```python
from build123d import *

# Parameters (mm, degrees)
F0_R     = 6
F1_DEPTH = 2
F2_R     = 2.5
F3_DEPTH = 1
F4_W     = 2.0085166757
F4_H     = 2
F5_DEPTH = 12.5
F6_R     = 0.5


with BuildPart() as f1:
    # F0 (on Front) → F1 (new body)
    with BuildSketch(Plane.XZ):
        Circle(F0_R)
    extrude(amount=F1_DEPTH)

    # F2 (on face) → F3 (cut)
    with BuildSketch(Plane(origin=(0, 0, 0), x_dir=(-1, 0, 0), z_dir=(0, 1, 0))):
        Circle(F2_R)
    extrude(amount=-F3_DEPTH, mode=Mode.SUBTRACT)

    # F4 (on Right) → F5 (cut, symmetric)
    with BuildSketch(Plane.YZ):
        with Locations((-2.1042583379, 0)):
            Rectangle(F4_W, F4_H)
    extrude(amount=F5_DEPTH, both=True, mode=Mode.SUBTRACT)

    # F6
    f6_edges = [f1.edges().sort_by_distance(p)[0] for p in [
        (0, -2, -6),
        (0, -2, 6),
    ]]
    fillet(f6_edges, radius=F6_R)


solid = f1.part
```
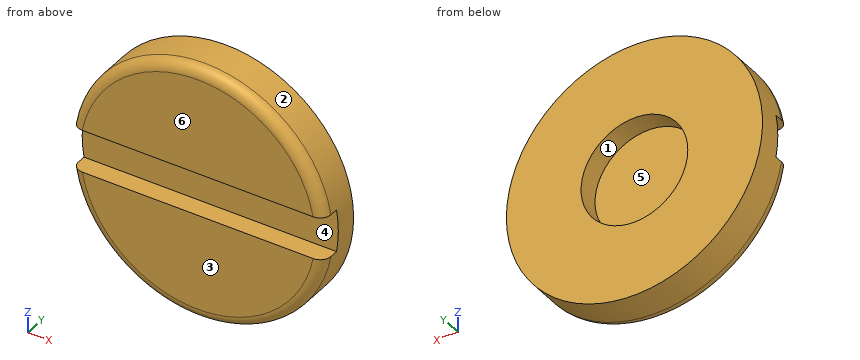
Work out the finished part from the listing and answer in its coordinate system (mm). Face numbers are marked on the shaded views. A direction names the side the tool comes from. Coordinates: 2 decimals unless noted, no trailing zeros. Loops run counter-clockwise (first coordinate to the right, second up) from the corner with the lowest first, then second, coordinate; pieces in that order, holes last. Notation, with made-up numbers: M 7.25,43 L 38.25,43 A31 cw 38.25,76 Z; hole C 9.25,55.5 d2. An arc over 180 degrees is marked long. Use CSV: the item, a comma, the result in double quotes. Start each with the question number.
(1) For the marked faces 4, 5 and 6, determine the directions among +Z, -Z, +X, -X, +Y, -Y from which every point of the face is accessible in a straight line to the end or side of a thin tool.
(2) Find section C-C, the plane y = -0.85. Give the vertices of the cut face in (x, z), then the cut area to 3 significant figures.
(3) Find section A-A, the plane x = 0. Give the vertices of the cut face in (y, z).
(4) Given pin 1 Ø1.6 at (x, z) = (-2, 0.5) entering from -Y; pin 2 Ø0.5 at (x, y) = (0.5, -1.5) entering from +Z; pin 3 Ø4 at (x, z) = (0, 0) entering from +Y, each flat-ended and moving along its own axis, determine where each tip first touches the part or whether it passes through.
(5) Find section D-D, the plane y = -1.7. Give the vertices of the cut face in (x, z).
(6) For a pull along Z with two mould halves and no side action, classify the marked faces 1, 2 and 3 as +Z half, -Z half, draft (parallel to the pull), parting line (faces both ways), or undercut.
(7) Consider line 1 (Z direction, x = 0, y = -0.3); line 2 (Z direction, x = 3, y = -1.8); line 3 (Y direction, x = -5.25, z = -0.5). Determine where each line is inside the solid, lowest interval first.
(8) Find section B-B, the plane z = 0. Give the vertices of the cut face in (x, y).
Recorded:
1,face 4,"+X, -X, -Y"
1,face 5,"+Y"
1,face 6,"+Z, -Z, +X, -X, -Y"
2,outline,"C 0,0 d12; hole C 0,0 d5"
2,area,"93.5 mm^2"
3,outline,"M -2,-5.5 A0.5 ccw -1.5,-6 L 0,-6 L 0,-2.5 L -1,-2.5 L -1,2.5 L 0,2.5 L 0,6 L -1.5,6 A0.5 ccw -2,5.5 L -2,1 L -1.1,1 L -1.1,-1 L -2,-1 Z"
4,pin 1,"stops at y = -2"
4,pin 2,"stops at z = 5.99"
4,pin 3,"stops at y = -1"
5,outline,"M -5.87,-1 A5.96 ccw 5.87,-1 Z; M -5.87,1 L 5.87,1 A5.96 ccw Z"
6,face 1,"undercut"
6,face 2,"parting line"
6,face 3,"draft"
7,line 1,"z = -6 to -2.5, 2.5 to 6"
7,line 2,"z = -5.08 to -1, 1 to 5.08"
7,line 3,"y = -1.1 to 0"
8,outline,"M -6,-1.1 L 6,-1.1 L 6,0 L 2.5,0 L 2.5,-1 L -2.5,-1 L -2.5,0 L -6,0 Z"
